from build123d import *

# Parameters (mm, degrees)
F0_R     = 6.477
F1_DEPTH = 30.48
F2_R     = 5.207
F3_DEPTH = 30.48
F5_W     = 10.922
F5_H     = 30.48
F6_DEPTH = 3.175
F7_R     = 1.27
F8_DEPTH = 2.38125


with BuildPart() as f1:
    # F0 (on Front) → F1 (new body)
    with BuildSketch(Plane.XZ):
        Circle(F0_R)
    extrude(amount=F1_DEPTH)

    # F2 (on face) → F3 (cut, through all)
    with BuildSketch(Plane(origin=(0, 0, 0), x_dir=(-1, 0, 0), z_dir=(0, 1, 0))):
        Circle(F2_R)
    extrude(amount=-F3_DEPTH, mode=Mode.SUBTRACT)

    # F5 (on offset) → F6 (join)
    with BuildSketch(Plane.XY.offset(-5.207)):
        with Locations((0, -15.24)):
            Rectangle(F5_W, F5_H)
    extrude(amount=-F6_DEPTH)

    # F7 (on face) → F8 (cut)
    with BuildSketch(Plane(origin=(0, 0, -8.382), x_dir=(1, 0, 0), z_dir=(0, 0, -1))):
        with BuildLine():
            Line((3.569046, 6.647212), (2.050303, 24.884939))
            ThreePointArc((2.050303, 24.884939), (0, 26.7716), (-2.050303, 24.884939))
            Line((-2.050303, 24.884939), (-3.569046, 6.647212))
            ThreePointArc((-3.569046, 6.647212), (0, 2.7686), (3.569046, 6.647212))
        make_face()
        with Locations((0, 6.35)):
            Circle(F7_R, mode=Mode.SUBTRACT)
        with Locations((0, 6.35)):
            Circle(F7_R)
    extrude(amount=-F8_DEPTH, mode=Mode.SUBTRACT)


solid = f1.part
Build history of the part. All positions in model axes, mm. A direction names the side the tool comes from. Round coordinates to 2 decimals unless told otherwise and drop trailing zeros. Write each loop counter-clockwise with the first axis right and the second up, starting at its lowest first coordinate (ties: lowest second). Pieces come first, ordered by that corner, then holes. Notation, with made-up numbers: M 22.25,48.25 L 53.25,48.25 A15 ccw 53.25,54.25 Z; hole C 62.25,-11 d5. An arc over 180 degrees is marked long. Answer as a JSON object with one key per item and string values. Group by question number.
(1) Cut at D-D (z = -2). Give the cut face in (x, y).
(2) Cut at B-B (x = 0). Give the cut face in (y, z), and give its area (3 significant figures).
(3) Which spindle directions (+Z, -Z, +X, -X, +Y, -Y) get a long thin tool onto all of the face, cutting with end or side? Do faces 5 (the flat face through (5.461, -15, -7)), 6 (the flat face through (0, -30.48, -6)), 7 (the cylindrical face through (-0.08, -2.77, -7.21)). Say none if no direction does.
(4) Cut at A-A (y = -6.35). Give the cut face in (x, z).
(5) Drill centre lines: L1, parallel to X at y = -6.35, z = -6.9; L2, parallel to Y at x = 0, z = -7.55; L3, parallel to X at y = -13, z = 0. Where is each one in solid material? Low to high.
(6) Flat gauge pins, fed straight in: pin 1 (2 mm diameter, centred on y = -19, z = -5, fed in from -X); pin 2 (6 mm diameter, centred on y = -4, z = -6, fed in from +X); pin 3 (0.8 mm diameter, centred on x = -4.5, y = -20, fed in from +Z). Where does each tip first touch, or does it go through?
(7) Cut at C-C (z = 0). Give the cut face in (x, y), and give its area (3 significant figures).
(8) Mould opens along X. For faces 1 (the flat face through (-4, -15, -8.382)), 2 (the flat face through (0, -15, -6.001)), 3 (the flat face through (-5.461, -15, -7)), 4 (the flat face through (2.82, -15.64, -7.21)) say: pulls with the +X half, pulls with the -X half, needs draft (parallel to the pull), parting line crosses it, or undercut.
Responses:
{
 "1": {"outline": "M -6.16,-30.48 L -4.81,-30.48 L -4.81,0 L -6.16,0 Z; M 4.81,-30.48 L 6.16,-30.48 L 6.16,0 L 4.81,0 Z"},
 "2": {"outline": "M -30.48,-8.38 L -26.77,-8.38 L -26.77,-6 L -2.77,-6 L -2.77,-8.38 L 0,-8.38 L 0,-5.21 L -30.48,-5.21 Z; M -30.48,5.21 L 0,5.21 L 0,6.48 L -30.48,6.48 Z", "area": "78.3 mm2"},
 "3": {"face 5": "-Z, +X, +Y, -Y", "face 6": "+Z, -Z, +X, -X, -Y", "face 7": "-Z"},
 "4": {"outline": "M -5.46,-8.38 L -3.58,-8.38 L -3.58,-6 L 3.58,-6 L 3.58,-8.38 L 5.46,-8.38 L 5.46,-5.21 L 3.85,-5.21 A6.48 ccw long -3.85,-5.21 L -5.46,-5.21 Z; hole C 0,0 d10.41"},
 "5": {"L1": "x = -5.46 to -3.58, 3.58 to 5.46", "L2": "y = -30.48 to -26.77, -2.77 to 0", "L3": "x = -6.48 to -5.21, 5.21 to 6.48"},
 "6": {"pin 1": "stops at x = -5.46", "pin 2": "stops at x = 5.74", "pin 3": "stops at z = 5.01"},
 "7": {"outline": "M -6.48,-30.48 L -5.21,-30.48 L -5.21,0 L -6.48,0 Z; M 5.21,-30.48 L 6.48,-30.48 L 6.48,0 L 5.21,0 Z", "area": "77.4 mm2"},
 "8": {"face 1": "needs draft", "face 2": "undercut", "face 3": "pulls with the -X half", "face 4": "undercut"}
}
